```python
from build123d import *

# Parameters (mm, degrees)
SKETCH_1_W                   = 33
SKETCH_1_H                   = 14.3
SKETCH_1_W_2                 = 29
SKETCH_1_H_2                 = 10.3
EXTRUDE_2_DEPTH              = 36
SKETCH_2_W                   = 33
SKETCH_2_H                   = 14.3
SKETCH_2_RX                  = 14.5
SKETCH_2_RY                  = 5.15
EXTRUDE_3_DEPTH              = 3
PATTERN_LINEAR_1_OUTLINE_W   = 33
PATTERN_LINEAR_1_OUTLINE_H   = 41.3
PATTERN_LINEAR_1_OUTLINE_W_2 = 29
PATTERN_LINEAR_1_OUTLINE_H_2 = 10.3
PATTERN_LINEAR_1_DEPTH       = 39
PATTERN_START                = 36
PATTERN_LINEAR_1_2_DEPTH     = 3


with BuildPart() as part:
    # Sketch 1 → Extrude 2 (new body)
    with BuildSketch(Plane(origin=(0, 0, 0), x_dir=(1, 0, 0), z_dir=(0, 1, 0))):
        Rectangle(SKETCH_1_W, SKETCH_1_H)
        Rectangle(SKETCH_1_W_2, SKETCH_1_H_2, mode=Mode.SUBTRACT)
    extrude(amount=EXTRUDE_2_DEPTH)

    # Sketch 2 → Extrude 3 (add)
    with BuildSketch(Plane(origin=(0, 36, 0), x_dir=(1, 0, 0), z_dir=(0, 1, 0))):
        Rectangle(SKETCH_2_W, SKETCH_2_H)
        with Locations(Location((0, 0), (0, 0, 0))):
            Ellipse(SKETCH_2_RX, SKETCH_2_RY, mode=Mode.SUBTRACT)
    extrude(amount=EXTRUDE_3_DEPTH)

    # Pattern Linear 1: read off the stored shape, not the designer's step
    # Pattern Linear 1 outline → Pattern Linear 1 (add)
    with BuildSketch(Plane(origin=(0, 0, 0), x_dir=(1, 0, 0), z_dir=(0, 1, 0))):
        with Locations((0, -13.5)):
            Rectangle(PATTERN_LINEAR_1_OUTLINE_W, PATTERN_LINEAR_1_OUTLINE_H)
        with Locations((0, -27)):
            Rectangle(PATTERN_LINEAR_1_OUTLINE_W_2, PATTERN_LINEAR_1_OUTLINE_H_2, mode=Mode.SUBTRACT)
        with Locations((0, -13.5)):
            Rectangle(PATTERN_LINEAR_1_OUTLINE_W_2, PATTERN_LINEAR_1_OUTLINE_H_2, mode=Mode.SUBTRACT)
        Rectangle(PATTERN_LINEAR_1_OUTLINE_W_2, PATTERN_LINEAR_1_OUTLINE_H_2, mode=Mode.SUBTRACT)
    extrude(amount=PATTERN_LINEAR_1_DEPTH)

    # Pattern Linear 1 2 outline → Pattern Linear 1 2 (add)
    with BuildSketch(Plane(origin=(0, 0, 0), x_dir=(1, 0, 0), z_dir=(0, 1, 0)).offset(PATTERN_START)):
        with BuildLine():
            Line((0, -32.15), (14.5, -32.15))
            Line((14.5, -32.15), (14.5, -27))
            add(Edge.make_bspline(
                [(0, -32.15), (14.5, -32.15), (14.5, -27)],
                knots=[4.71238898, 4.71238898, 4.71238898, 6.283185307, 6.283185307, 6.283185307], degree=2, weights=[1, 0.707106781, 1]))
        make_face()
        with BuildLine():
            add(Edge.make_bspline(
                [(14.5, -27), (14.5, -21.85), (0, -21.85)],
                knots=[0, 0, 0, 1.570796327, 1.570796327, 1.570796327], degree=2, weights=[1, 0.707106781, 1]))
            Line((14.5, -27), (14.5, -21.85))
            Line((14.5, -21.85), (0, -21.85))
        make_face()
        with BuildLine():
            Line((-14.5, -32.15), (0, -32.15))
            add(Edge.make_bspline(
                [(-14.5, -27), (-14.5, -32.15), (0, -32.15)],
                knots=[3.141592654, 3.141592654, 3.141592654, 4.71238898, 4.71238898, 4.71238898], degree=2, weights=[1, 0.707106781, 1]))
            Line((-14.5, -27), (-14.5, -32.15))
        make_face()
        with BuildLine():
            add(Edge.make_bspline(
                [(0, -21.85), (-14.5, -21.85), (-14.5, -27)],
                knots=[1.570796327, 1.570796327, 1.570796327, 3.141592654, 3.141592654, 3.141592654], degree=2, weights=[1, 0.707106781, 1]))
            Line((0, -21.85), (-14.5, -21.85))
            Line((-14.5, -21.85), (-14.5, -27))
        make_face()
        with BuildLine():
            Line((0, -18.65), (14.5, -18.65))
            Line((14.5, -18.65), (14.5, -13.5))
            add(Edge.make_bspline(
                [(0, -18.65), (14.5, -18.65), (14.5, -13.5)],
                knots=[4.71238898, 4.71238898, 4.71238898, 6.283185307, 6.283185307, 6.283185307], degree=2, weights=[1, 0.707106781, 1]))
        make_face()
        with BuildLine():
            add(Edge.make_bspline(
                [(14.5, -13.5), (14.5, -8.35), (0, -8.35)],
                knots=[0, 0, 0, 1.570796327, 1.570796327, 1.570796327], degree=2, weights=[1, 0.707106781, 1]))
            Line((14.5, -13.5), (14.5, -8.35))
            Line((14.5, -8.35), (0, -8.35))
        make_face()
        with BuildLine():
            Line((-14.5, -18.65), (0, -18.65))
            add(Edge.make_bspline(
                [(-14.5, -13.5), (-14.5, -18.65), (0, -18.65)],
                knots=[3.141592654, 3.141592654, 3.141592654, 4.71238898, 4.71238898, 4.71238898], degree=2, weights=[1, 0.707106781, 1]))
            Line((-14.5, -13.5), (-14.5, -18.65))
        make_face()
        with BuildLine():
            add(Edge.make_bspline(
                [(0, -8.35), (-14.5, -8.35), (-14.5, -13.5)],
                knots=[1.570796327, 1.570796327, 1.570796327, 3.141592654, 3.141592654, 3.141592654], degree=2, weights=[1, 0.707106781, 1]))
            Line((0, -8.35), (-14.5, -8.35))
            Line((-14.5, -8.35), (-14.5, -13.5))
        make_face()
    extrude(amount=PATTERN_LINEAR_1_2_DEPTH)


solid = part.part
```
Input: part model. Units: mm. Frame: model coordinates. A direction names the side the tool comes from. Coordinates: 2 decimals unless noted, no trailing zeros. Write each loop counter-clockwise with the first axis right and the second up, starting at its lowest first coordinate (ties: lowest second). Pieces come first, ordered by that corner, then holes.
1) Material intervals for line 1 along Z through (x, y) = (0.5, 2); line 2 along X through (y, z) = (17.5, 2); line 3 along Z through (x, y) = (13, 36.5), sorted ascending.
2) Section A-A on y = 10.5. Output: boundary loops of the cut face in (x, z).
3) Pin query (flat end, axial travel): pin 1 Ø5.5 at (x, z) = (-10, 2) entering from -Y. Return the tip coordinate at first contact, or that it passes through.
4) Mould query, pull axis X, two halves, no side actions, for faces 1 (the flat face through (-14.5, 18, 27)), 2 (the flat face through (-16.5, 19, 14)), 3 (the flat face through (16.5, 19, 14)), 4 (the flat face through (-8, 39, 9)). Classes: pulls with the +X half, pulls with the -X half, needs draft (parallel to the pull), parting line crosses it, or undercut.
5) Section B-B on x = 5. State how many separate pieces and enclosed holes the cut face has, and give its area (3 significant figures).
6) Set-up query: faces 5 (the flat face through (0, 19, -7.15)), 6 (the flat face through (0, 18, -5.15)). Return all of +Z, -Z, +X, -X, +Y, -Y with unobstructed straight access to the full face (end or side cutting, diameter ignored); none if empty.
Check result:
1. line 1: z = -7.15 to -5.15, 5.15 to 8.35, 18.65 to 21.85, 32.15 to 34.15
1. line 2: x = -16.5 to -14.5, 14.5 to 16.5
1. line 3: z = -7.15 to -2.28, 2.28 to 11.22, 15.78 to 24.72, 29.28 to 34.15
2. outline: (-16.5, -7.15) - (16.5, -7.15) - (16.5, 34.15) - (-16.5, 34.15) - close; hole (-14.5, -5.15) - (14.5, -5.15) - (14.5, 5.15) - (-14.5, 5.15) - close; hole (-14.5, 8.35) - (14.5, 8.35) - (14.5, 18.65) - (-14.5, 18.65) - close; hole (-14.5, 21.85) - (14.5, 21.85) - (14.5, 32.15) - (-14.5, 32.15) - close
3. pin 1: stops at y = 36
4. face 1: undercut
4. face 2: pulls with the -X half
4. face 3: pulls with the +X half
4. face 4: needs draft
5. separate pieces: 4
5. enclosed holes: 0
5. area: 411 mm2
6. face 5: -Z, +X, -X, +Y, -Y
6. face 6: -Y
